For this review, take the finished solid that the model builds, in its own axes (mm). Give positions to 0.01 mm unless a question says otherwise; leave off trailing zeros. Order: outer loops, then holes, each group sorted by start corner. A loop starts at its lowest first (then second) coordinate and runs counter-clockwise, first axis right, second up.
from build123d import *

# Parameters (mm, degrees)
SKETCH1_R           = 50
SKETCH1_R_2         = 1.55
SKETCH1_W           = 30.561449232
SKETCH1_H           = 6
BOSS_EXTRUDE2_DEPTH = 2
FILLET1_R           = 3


with BuildPart() as part:
    # Sketch1 → Boss-Extrude2 (new body)
    # profile 1 of 7: a face of its own
    with BuildSketch(Plane(origin=(0, 0, 0), x_dir=(1, 0, 0), z_dir=(0, 1, 0))):
        with Locations(Location((0, 0, 0), (0, 0, 270))):
            Circle(SKETCH1_R)
        Polygon((-28.355339059, 15.280724616), (-28.355339059, 28.355339059), (-15.280724616, 28.355339059), (-15.280724616, 37.17766953), (0, 46), (15.280724616, 37.17766953), (15.280724616, 28.355339059), (28.355339059, 28.355339059), (28.355339059, 15.280724616), (37.17766953, 15.280724616), (46, 0), (37.17766953, -15.280724616), (28.355339059, -15.280724616), (28.355339059, -28.355339059), (15.280724616, -28.355339059), (15.280724616, -37.17766953), (0, -46), (-15.280724616, -37.17766953), (-15.280724616, -28.355339059), (-28.355339059, -28.355339059), (-28.355339059, -15.280724616), (-37.17766953, -15.280724616), (-46, 0), (-37.17766953, 15.280724616), align=None, mode=Mode.SUBTRACT)
    # profile 2 of 7: a face of its own
    with BuildSketch(Plane(origin=(0, 0, 0), x_dir=(1, 0, 0), z_dir=(0, 1, 0))):
        Polygon((28.355339059, -28.355339059), (28.355339059, -15.280724616), (22.355339059, -15.280724616), (22.355339059, -22.355339059), (15.280724616, -22.355339059), (15.280724616, -28.355339059), align=None)
        with Locations(Location((25.355339059, -25.355339059, 0), (0, 0, 270))):
            Circle(SKETCH1_R_2, mode=Mode.SUBTRACT)
    # profile 3 of 7: a face of its own
    with BuildSketch(Plane(origin=(0, 0, 0), x_dir=(1, 0, 0), z_dir=(0, 1, 0))):
        Polygon((-22.355339059, -15.280724616), (-28.355339059, -15.280724616), (-28.355339059, -28.355339059), (-15.280724616, -28.355339059), (-15.280724616, -22.355339059), (-22.355339059, -22.355339059), align=None)
        with Locations(Location((-25.355339059, -25.355339059, 0), (0, 0, 270))):
            Circle(SKETCH1_R_2, mode=Mode.SUBTRACT)
    # profile 4 of 7: a face of its own
    with BuildSketch(Plane(origin=(0, 0, 0), x_dir=(1, 0, 0), z_dir=(0, 1, 0))):
        Polygon((-15.280724616, 28.355339059), (-28.355339059, 28.355339059), (-28.355339059, 15.280724616), (-22.355339059, 15.280724616), (-22.355339059, 22.355339059), (-15.280724616, 22.355339059), align=None)
        with Locations(Location((-25.355339059, 25.355339059, 0), (0, 0, 270))):
            Circle(SKETCH1_R_2, mode=Mode.SUBTRACT)
    # profile 5 of 7: a face of its own
    with BuildSketch(Plane(origin=(0, 0, 0), x_dir=(1, 0, 0), z_dir=(0, 1, 0))):
        Polygon((28.355339059, 28.355339059), (15.280724616, 28.355339059), (15.280724616, 22.355339059), (22.355339059, 22.355339059), (22.355339059, 15.280724616), (28.355339059, 15.280724616), align=None)
        with Locations(Location((25.355339059, 25.355339059, 0), (0, 0, 270))):
            Circle(SKETCH1_R_2, mode=Mode.SUBTRACT)
    # profile 6 of 7: a face of its own
    with BuildSketch(Plane(origin=(0, 0, 0), x_dir=(1, 0, 0), z_dir=(0, 1, 0))):
        with Locations((0, 25.355339059)):
            Rectangle(SKETCH1_W, SKETCH1_H)
    # profile 7 of 7: a face of its own
    with BuildSketch(Plane(origin=(0, 0, 0), x_dir=(1, 0, 0), z_dir=(0, 1, 0))):
        Polygon((-15.280724616, 37.17766953), (-15.280724616, 28.355339059), (15.280724616, 28.355339059), (15.280724616, 37.17766953), (0, 46), align=None)
    extrude(amount=BOSS_EXTRUDE2_DEPTH)

    # Fillet1
    fillet1_edges = [part.edges().sort_by_distance(p)[0] for p in [
        (-22.355339059, 1, -15.280724616),
        (-37.17766953, 1, -15.280724616),
        (-46, 1, 0),
        (-37.17766953, 1, 15.280724616),
        (-22.355339059, 1, 15.280724616),
        (-22.355339059, 1, 22.355339059),
        (-15.280724616, 1, 22.355339059),
        (-15.280724616, 1, 37.17766953),
        (0, 1, 46),
        (15.280724616, 1, 37.17766953),
        (22.355339059, 1, 22.355339059),
        (37.17766953, 1, 15.280724616),
        (46, 1, 0),
        (37.17766953, 1, -15.280724616),
        (22.355339059, 1, -22.355339059),
        (-22.355339059, 1, -22.355339059),
    ]]
    fillet(fillet1_edges, radius=FILLET1_R)


solid = part.part
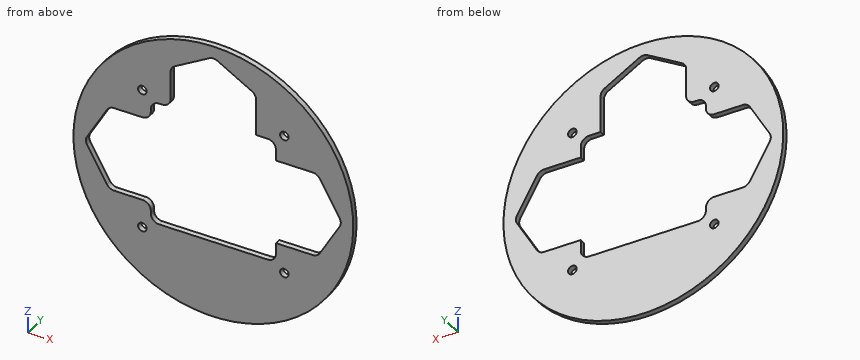
1) To check wall thickness, follow line 1 (X direction, y = 1.35, z = 32); line 2 (Z direction, x = 8, y = 1.1); line 3 (Z direction, x = 33, y = 0.25). State the ranges of each line that lie inside material, in increasing order.
Answer sheet:
line 1: x = -38.42 to -15.28, 15.28 to 38.42
line 2: z = -49.36 to -22.36, 41.38 to 49.36
line 3: z = -37.56 to -15.28, 15.28 to 37.56
2) We need section D-D on z = -35. Give the boundary of the cut face in (x, y), then the cut area to 3 significant figures.
Answer sheet:
outline: (-35.71, 0) - (35.71, 0) - (35.71, 2) - (-35.71, 2) - close
area: 143 mm2
3) Clearance check with flat-ended pins moving along their axes: pin 1 (0.6 mm diameter, centred on y = 1, z = 31.5, fed in from +X); pin 2 (1 mm diameter, centred on x = 7, y = 1, fed in from +Z); pin 3 (1.2 mm diameter, centred on x = -18.5, y = 1.5, fed in from -Z); pin 4 (2.5 mm diameter, centred on x = -25.36, z = 25.36, fed in from -Y). State where each tip first meets the part, or that it passes through.
Answer sheet:
pin 1: stops at x = 39.07
pin 2: stops at z = 49.58
pin 3: stops at z = -46.69
pin 4: passes through
4) We need section A-A on x = 0. Give the boundary of the cut face in (y, z), then the cut area to 3 significant figures.
Answer sheet:
outline: (0, -50) - (2, -50) - (2, -22.36) - (0, -22.36) - close; (0, 45.54) - (2, 45.54) - (2, 50) - (0, 50) - close
area: 64.2 mm2
5) We need section C-C on y = 1.1. Count the separate pieces of the cut face and the enclosed holes in it, then the cut area to 3 significant figures.
Answer sheet:
separate pieces: 1
enclosed holes: 5
area: 4,070 mm2
6) We need section B-B on z = 0. Give the boundary of the cut face in (x, y), then the cut area to 3 significant figures.
Answer sheet:
outline: (-50, 0) - (-45.54, 0) - (-45.54, 2) - (-50, 2) - close; (45.54, 0) - (50, 0) - (50, 2) - (45.54, 2) - close
area: 17.9 mm2
